Build history of the part. All positions in model axes, mm. A direction names the side the tool comes from. Coordinates: 2 decimals unless noted, no trailing zeros. Order: outer loops, then holes, each group sorted by start corner. A loop starts at its lowest first (then second) coordinate and runs counter-clockwise, first axis right, second up. Notation, with made-up numbers: (-6, 69) - (51, 69) arc R29 cw to (51, 102) - close; hole circle Ø8 at (-8.5, 50). An arc over 180 degrees is marked (long way). One line per item, written item: value.
Autodesk Inventor part; units mm, degrees
ref_plane "YZ Plane" through (0, 0, 0) normal (1, 0, 0) x (0, 1, 0)
ref_plane "XZ Plane" through (0, 0, 0) normal (0, 1, 0) x (-1, 0, 0)
ref_plane "XY Plane" through (0, 0, 0) normal (0, 0, 1) x (1, 0, 0)
sketch "Sketch1" plane through (0, 0, 0) normal (0, 0, 1) x (1, 0, 0)
  circle A0 centre (0, 0) radius 8
  line L0 (0, 0) -> (16, 0) construction
  arc A1 (11.746, 0.9) -> (7.746, 2) centre (5.8068, -12.8741) ccw
  arc A2 (7.746, -2) -> (11.746, -0.9) centre (5.8068, 12.8741) ccw
  arc A3 (7.746, -2) -> (7.746, 2) centre (0, 0) ccw
  arc A4 (11.746, -0.9) -> (11.746, 0.9) centre (-8.2338, 0) ccw
  arc A5 (9.3948, 7.1075) -> (5.435, 5.8703) centre (11.8453, -7.691) ccw
  arc A6 (10.3679, 5.5932) -> (9.3948, 7.1075) centre (-6.9267, -4.4515) ccw
  arc A7 (7.5976, 2.5053) -> (10.3679, 5.5932) centre (-2.0753, 13.9698) ccw
  arc A8 (7.5976, 2.5053) -> (5.435, 5.8703) centre (0, 0) ccw
  arc A9 (4.0608, 11.0584) -> (1.3985, 7.8768) centre (14.123, -0.066) ccw
  arc A10 (5.6981, 10.3106) -> (4.0608, 11.0584) centre (-3.4204, -7.4897) ccw
  arc A11 (5.0371, 6.2151) -> (5.6981, 10.3106) centre (-9.2985, 10.6302) ccw
  arc A12 (5.0371, 6.2151) -> (1.3985, 7.8768) centre (0, 0) ccw
  arc A13 (-2.5625, 11.4983) -> (-3.082, 7.3825) centre (11.9167, 7.5799) ccw
  arc A14 (-0.7808, 11.7545) -> (-2.5625, 11.4983) centre (1.1718, -8.15) ccw
  arc A15 (0.8773, 7.9518) -> (-0.7808, 11.7545) centre (-13.5695, 3.9155) ccw
  arc A16 (0.8773, 7.9518) -> (-3.082, 7.3825) centre (0, 0) ccw
  arc A17 (-8.3721, 8.2876) -> (-6.584, 4.5443) centre (5.927, 12.8193) ccw
  arc A18 (-7.0118, 9.4664) -> (-8.3721, 8.2876) centre (5.392, -6.2227) ccw
  arc A19 (-3.561, 7.1637) -> (-7.0118, 9.4664) centre (-13.5323, -4.0423) ccw
  arc A20 (-3.561, 7.1637) -> (-6.584, 4.5443) centre (0, 0) ccw
  arc A21 (-11.5237, 2.4457) -> (-7.9957, 0.2633) centre (-1.9446, 13.9886) ccw
  arc A22 (-11.0166, 4.1728) -> (-11.5237, 2.4457) centre (7.9002, -2.3197) ccw
  arc A23 (-6.8687, 4.1013) -> (-11.0166, 4.1728) centre (-9.1987, -10.7167) ccw
  arc A24 (-6.8687, 4.1013) -> (-7.9957, 0.2633) centre (0, 0) ccw
  arc A25 (-11.0166, -4.1728) -> (-6.8687, -4.1013) centre (-9.1987, 10.7167) ccw
  arc A26 (-11.5237, -2.4457) -> (-11.0166, -4.1728) centre (7.9002, 2.3197) ccw
  arc A27 (-7.9957, -0.2633) -> (-11.5237, -2.4457) centre (-1.9446, -13.9886) ccw
  arc A28 (-7.9957, -0.2633) -> (-6.8687, -4.1013) centre (0, 0) ccw
  arc A29 (-7.0118, -9.4664) -> (-3.561, -7.1637) centre (-13.5323, 4.0423) ccw
  arc A30 (-8.3721, -8.2876) -> (-7.0118, -9.4664) centre (5.392, 6.2227) ccw
  arc A31 (-6.584, -4.5443) -> (-8.3721, -8.2876) centre (5.927, -12.8193) ccw
  arc A32 (-6.584, -4.5443) -> (-3.561, -7.1637) centre (0, 0) ccw
  arc A33 (-0.7808, -11.7545) -> (0.8773, -7.9518) centre (-13.5695, -3.9155) ccw
  arc A34 (-2.5625, -11.4983) -> (-0.7808, -11.7545) centre (1.1718, 8.15) ccw
  arc A35 (-3.082, -7.3825) -> (-2.5625, -11.4983) centre (11.9167, -7.5799) ccw
  arc A36 (-3.082, -7.3825) -> (0.8773, -7.9518) centre (0, 0) ccw
  arc A37 (5.6981, -10.3106) -> (5.0371, -6.2151) centre (-9.2985, -10.6302) ccw
  arc A38 (4.0608, -11.0584) -> (5.6981, -10.3106) centre (-3.4204, 7.4897) ccw
  arc A39 (1.3985, -7.8768) -> (4.0608, -11.0584) centre (14.123, 0.066) ccw
  arc A40 (1.3985, -7.8768) -> (5.0371, -6.2151) centre (0, 0) ccw
  arc A41 (10.3679, -5.5932) -> (7.5976, -2.5053) centre (-2.0753, -13.9698) ccw
  arc A42 (9.3948, -7.1075) -> (10.3679, -5.5932) centre (-6.9267, 4.4515) ccw
  arc A43 (5.435, -5.8703) -> (9.3948, -7.1075) centre (11.8453, 7.691) ccw
  arc A44 (5.435, -5.8703) -> (7.5976, -2.5053) centre (0, 0) ccw
  point P0 (11.7662, 0)
  point P1 (9.8984, 6.3613)
  point P2 (4.8879, 10.7029)
  point P3 (-1.6745, 11.6465)
  point P4 (-7.7052, 8.8923)
  point P5 (-11.2896, 3.3149)
  point P6 (-11.2896, -3.3149)
  point P7 (-7.7052, -8.8923)
  point P8 (-1.6745, -11.6465)
  point P9 (4.8879, -10.7029)
  point P10 (9.8984, -6.3613)
  dimension "d0" = 16
  dimension "d1" = 16
  dimension "d2" = 15
  dimension "d3" = 4
  dimension "d4" = 2
  dimension "d6" = 1.8
  dimension "d15" = 20
  dimension "d18" = 360
extrude "Extrusion1" add sketch "Sketch1" along normal blind 15
sketch "Sketch2" plane through (0, 0, 15) normal (0, 0, 1) x (1, 0, 0)
  circle A0 centre (0, 0) radius 3
  circle A1 centre (0, 0) radius 8
  dimension "d22" = 6
  dimension "d23" = 16
extrude "Extrusion2" add sketch "Sketch2" along normal blind 10
sketch "Sketch3" plane through (0, 0, 25) normal (0, 0, 1) x (1, 0, 0)
  circle A0 centre (0, 0) radius 3
extrude "Extrusion3" cut sketch "Sketch3" against normal through all
sketch "Sketch4" plane through (0, 0, 0) normal (1, 0, 0) x (0, 1, 0)
  circle A0 centre (0, 19) radius 1.5
  line L0 (8, 25) -> (-8, 25)
  point P0 (0, 0)
  dimension "d28" = 3
  dimension "d29" = 6
extrude "Extrusion4" cut sketch "Sketch4" along normal through all
properties part number "Motor Gear" material "ABS Plastic"
1. Band-saw the part on C-C, the plane x = -6. Give the cut face in (y, z), and give its area (3 significant figures).
Values found:
outline: (-8.93, 0) - (8.93, 0) - (8.93, 15) - (5.29, 15) - (5.29, 25) - (-5.29, 25) - (-5.29, 15) - (-8.93, 15) - close
area: 374 mm2
2. Flat gauge pins, fed straight in: P1, Ø1.2, axis at x = -9.5, y = 3, coming from the +Z side; P2, Ø2, axis at y = 6, z = 11.5, coming from the +X side; P3, Ø1.8, axis at y = 0, z = 19, coming from the -X side. Where does each tip first touch, or does it go through?
Values found:
P1: stops at z = 15
P2: stops at x = 10.37
P3: stops at x = -8
3. Band-saw the part on D-D, the plane z = 19. Give the cut face in (x, y).
Values found:
outline: (2.6, -1.5) arc R3 cw (long way) to (2.6, 1.5) - (7.86, 1.5) arc R8 ccw (long way) to (7.86, -1.5) - close
4. Probe line 1 along Y through (x, z) = (0, 18); line 2 along Y through (x, z) = (8.25, 7.25); line 3 along Z through (x, y) = (5.2, 0). List the from-to ranges inside material, lowest first.
Values found:
line 1: y = -8 to -3, 3 to 8
line 2: y = -6.87 to -3.09, -1.93 to 1.93, 3.09 to 6.87
line 3: z = 0 to 17.5, 20.5 to 25
5. Band-saw the part on A-A, the plane x = 0. Give the cut face in (y, z).
Values found:
outline: (-10.31, 0) - (-3, 0) - (-3, 25) - (-8, 25) - (-8, 15) - (-10.31, 15) - close; (3, 0) - (10.31, 0) - (10.31, 15) - (8, 15) - (8, 25) - (3, 25) - close
6. Band-saw the part on B-B, the plane x = 9.75. Give the cut face in (y, z), and give its area (3 significant figures).
Values found:
outline: (-6.59, 0) - (-4.74, 0) - (-4.74, 15) - (-6.59, 15) - close; (-1.6, 0) - (1.6, 0) - (1.6, 15) - (-1.6, 15) - close; (4.74, 0) - (6.59, 0) - (6.59, 15) - (4.74, 15) - close
area: 103 mm2
7. 3-axis set-ups, long thin cutter, end or side, ignore diameter. For faces 4 (the face through (9.756, 1.597, 7.395)), 5 (the face through (-7.62, -6.38, 7.4)), 6 (the face through (7.63, -2.4, 17.88)), 7 (the face through (3, -10, 7)): which of +Z, -Z, +X, -X, +Y, -Y reach the whole face in a straight line?
Values found:
face 4: +Z, -Z, +X
face 5: +Z, -Z, -X
face 6: +Z
face 7: +Z, -Z, -Y
8. Two-plate mould, pull along X, no slides. Class faces 1 (the face through (5.515, 8.269, 7.395)), 2 (the face through (8, -5, 15)), 3 (the face through (-7.696, -8.901, 7.395)): pulls with the +X half, pulls with the -X half, needs draft (parallel to the pull), parting line crosses it, or undercut.
Values found:
face 1: undercut
face 2: needs draft
face 3: pulls with the -X half
